from build123d import *

# Parameters (mm, degrees)
SKETCH_1_W       = 200
SKETCH_1_H       = 200
BACKGROUND_DEPTH = 1
LOGO_DEPTH       = 10
FILLET_R_R       = 1


with BuildPart() as part:
    # 草图1 → Background (new body)
    with BuildSketch(Plane.XY):
        with Locations((100, -100)):
            Rectangle(SKETCH_1_W, SKETCH_1_H)
    extrude(amount=BACKGROUND_DEPTH)

    # 草图2 → Logo (cut)
    with BuildSketch(Plane.XY.offset(1)):
        with BuildLine():
            Line((44, -45), (75.594408409, -45))
            Line((75.594408409, -45), (61.483495706, -30.889087297))
            ThreePointArc((61.483495706, -30.889087297), (61.483495706, -23.110912703), (69.261670299, -23.110912703))
            Line((69.261670299, -23.110912703), (91.150757595, -45))
            Line((91.150757595, -45), (108.849242405, -45))
            Line((108.849242405, -45), (130.738329701, -23.110912703))
            ThreePointArc((130.738329701, -23.110912703), (138.516504294, -23.110912703), (138.516504294, -30.889087297))
            Line((138.516504294, -30.889087297), (124.405591591, -45))
            Line((124.405591591, -45), (156, -45))
            ThreePointArc((156, -45), (174.384776311, -52.615223689), (182, -71))
            Line((182, -71), (182, -136))
            Line((182, -136), (163, -136))
            Line((163, -136), (163, -71))
            ThreePointArc((163, -71), (160.071067812, -63.928932188), (153, -61))
            Line((153, -61), (47, -61))
            ThreePointArc((47, -61), (39.928932188, -63.928932188), (37, -71))
            Line((37, -71), (18, -71))
            ThreePointArc((18, -71), (25.615223689, -52.615223689), (44, -45))
        make_face()
        with BuildLine():
            Line((44, -168), (51, -168))
            Line((51, -168), (51, -169))
            ThreePointArc((51, -169), (59.5, -177.5), (68, -169))
            Line((68, -169), (68, -168))
            Line((68, -168), (132, -168))
            Line((132, -168), (132, -169))
            ThreePointArc((132, -169), (140.5, -177.5), (149, -169))
            Line((149, -169), (149, -168))
            Line((149, -168), (156, -168))
            ThreePointArc((156, -168), (174.384776311, -160.384776311), (182, -142))
            Line((182, -142), (163, -142))
            ThreePointArc((163, -142), (160.071067812, -149.071067812), (153, -152))
            Line((153, -152), (47, -152))
            ThreePointArc((47, -152), (39.928932188, -149.071067812), (37, -142))
            Line((37, -142), (37, -77))
            Line((37, -77), (18, -77))
            Line((18, -77), (18, -142))
            ThreePointArc((18, -142), (25.615223689, -160.384776311), (44, -168))
        make_face()
        Polygon((47.51948306, -91.53578191), (80.51948306, -85.121231708), (83, -97.882385093), (50, -104.296935295), align=None)
        Polygon((119.48051694, -84.796316416), (152.48051694, -91.210866617), (150, -103.972020002), (117, -97.557469801), align=None)
        with BuildLine():
            Line((78, -126), (83.5, -123))
            add(Edge.make_bspline(
                [(83.5, -123), (91.450014857, -135.202864972), (100, -118.812493298)],
                knots=[0, 0, 0, 1, 1, 1], degree=2))
            add(Edge.make_bspline(
                [(116.5, -123), (108.549985143, -135.202864972), (100, -118.812493298)],
                knots=[0, 0, 0, 1, 1, 1], degree=2))
            Line((116.5, -123), (122, -126))
            add(Edge.make_bspline(
                [(122, -126), (112.840164848, -140.569491763), (100, -130.315373567)],
                knots=[0, 0, 0, 1, 1, 1], degree=2))
            add(Edge.make_bspline(
                [(78, -126), (87.159835152, -140.569491763), (100, -130.315373567)],
                knots=[0, 0, 0, 1, 1, 1], degree=2))
        make_face()
    extrude(amount=-LOGO_DEPTH, mode=Mode.SUBTRACT)

    # R
    fillet_r_edges = [part.edges().sort_by_distance(p)[0] for p in [
        (122, -126, 0.5),
        (116.5, -123, 0.5),
        (100, -118.812493298, 0.5),
        (78, -126, 0.5),
        (83.5, -123, 0.5),
        (117, -97.557469801, 0.5),
        (150, -103.972020002, 0.5),
        (152.48051694, -91.210866617, 0.5),
        (119.48051694, -84.796316416, 0.5),
        (50, -104.296935295, 0.5),
        (83, -97.882385093, 0.5),
        (80.51948306, -85.121231708, 0.5),
        (47.51948306, -91.53578191, 0.5),
        (163, -142, 0.5),
        (182, -142, 0.5),
        (182, -136, 0.5),
        (163, -136, 0.5),
        (18, -71, 0.5),
        (37, -71, 0.5),
        (37, -77, 0.5),
        (18, -77, 0.5),
    ]]
    fillet(fillet_r_edges, radius=FILLET_R_R)


solid = part.part
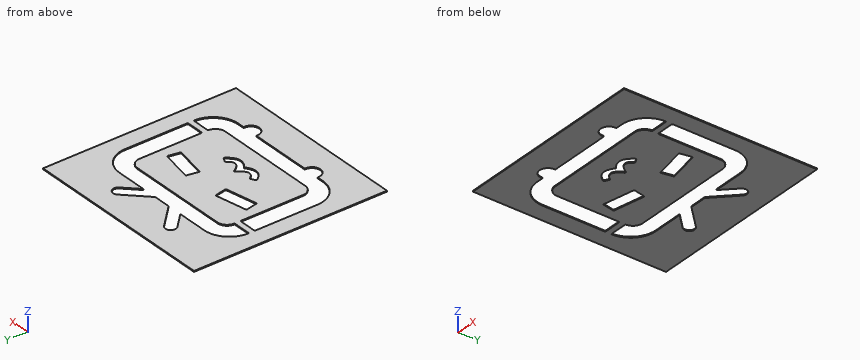
Geometry: final body of the model. Coordinates: model frame, mm. Give positions to 0.01 mm unless a question says otherwise; leave off trailing zeros. Write each loop counter-clockwise with the first axis right and the second up, starting at its lowest first coordinate (ties: lowest second). Pieces come first, ordered by that corner, then holes. Notation, with made-up numbers: (79, 14) -> (94, 14) arc R13 cw to (94, 28) -> close; hole circle Ø8 at (27, -20). An arc over 180 degrees is marked (long way). Answer in a Markdown table with one row per item.
(1) Section query B-B on y = -159.5. Return loops of the section in (x, z).
Answers below:
| item | result |
|---|---|
| outline | (0, 0) -> (24.77, 0) -> (24.77, 1) -> (0, 1) -> close; (175.23, 0) -> (200, 0) -> (200, 1) -> (175.23, 1) -> close |
(2) Pin query (flat end, axial travel): pin 1 (0.5 mm diameter, centred on x = 98.5, z = 0.5, fed in from +Y); pin 2 (1.5 mm diameter, centred on x = 61.5, y = -46, fed in from -Z). Return the tip coordinate at first contact, or that it passes through.
Answers below:
| item | result |
|---|---|
| pin 1 | y = 0 |
| pin 2 | through |
(3) Section query A-A on y = -116. Return loops of the section in (x, z), then the cut area to 3 significant figures.
Answers below:
| item | result |
|---|---|
| outline | (0, 0) -> (18, 0) -> (18, 1) -> (0, 1) -> close; (37, 0) -> (163, 0) -> (163, 1) -> (37, 1) -> close; (182, 0) -> (200, 0) -> (200, 1) -> (182, 1) -> close |
| area | 162 mm^2 |
(4) Section query D-D on y = -27. Return loops of the section in (x, z), then the cut area to 3 significant figures.
Answers below:
| item | result |
|---|---|
| outline | (0, 0) -> (59.87, 0) -> (59.87, 1) -> (0, 1) -> close; (73.15, 0) -> (126.85, 0) -> (126.85, 1) -> (73.15, 1) -> close; (140.13, 0) -> (200, 0) -> (200, 1) -> (140.13, 1) -> close |
| area | 173 mm^2 |
(5) Ray query, line 1 along Y through (x, z) = (46, 0.2); line 2 along Y through (x, z) = (33, 0.85); line 3 along Y through (x, z) = (57, 0.9). Return the intervals inside material, ascending. Write a range as [from, to].
Answers below:
| item | result |
|---|---|
| line 1 | [-200, -168], [-151.95, -61.05], [-45, 0] |
| line 2 | [-200, -165.56], [-77, -71], [-47.44, 0] |
| line 3 | [-200, -177.12], [-152, -102.94], [-89.69, -61], [-45, 0] |
(6) Section query C-C on z = 0.6. State how many separate pieces and enclosed holes the cut face has, then the cut area to 3 significant figures.
Answers below:
| item | result |
|---|---|
| separate pieces | 1 |
| enclosed holes | 5 |
| area | 29,900 mm^2 |
